Job drawing, mm, ordinate dimensions from the low corner. One solid piece. A direction names the side the tool comes from. Round coordinates to 2 decimals unless told otherwise and drop trailing zeros. Loops run counter-clockwise (first coordinate to the right, second up) from the corner with the lowest first, then second, coordinate; pieces in that order, holes last. Notation, with made-up numbers: M 78.25,-4.75 L 105.25,-4.75 A24 cw 105.25,13.25 Z; hole C 13.25,46.25 d5. An arc over 180 degrees is marked long. Use a Markdown table: item, result. Add a question column.
(1) Band-saw the part on C-C, the plane x = 44.5. Write the cut outline in (y, z), and give its area (3 significant figures).
(2) Band-saw the part on B-B, the plane y = 31. Write the cut outline in (x, z), and give its area (3 significant figures).
(3) Band-saw the part on D-D, the plane y = 59. Write the cut outline in (x, z).
(4) Which spindle directions (+Z, -Z, +X, -X, +Y, -Y) get a long thin tool onto all of the face, cutting with end or side? Do the marked faces 4, 5, 6 and 7. Say none if no direction does.
(5) Two-plate mould, pull along X, no slides. Class the marked faces 1, 2 and 3: released by +X, released by -X, zero draft, split by the parting line, or undercut.
(6) Flat gauge pins, fed straight in: P1, Ø10, axis at x = 17, z = 11, coming from the +Y side; P2, Ø1.5, axis at x = 27, y = 43, coming from the +Z side; P3, Ø12.5, axis at x = 35, z = 29.5, coming from the +Y side. Where does each tip first touch, or does it go through?
(7) Band-saw the part on A-A, the plane z = 42. Write the cut outline in (x, y).
(8) Wall check: L1, parallel to Y at x = 98.5, z = 44; L2, parallel to Y at x = 10.5, z = 35; L3, parallel to X at y = 28, z = 20. Give the ranges that are in metal, low to high.
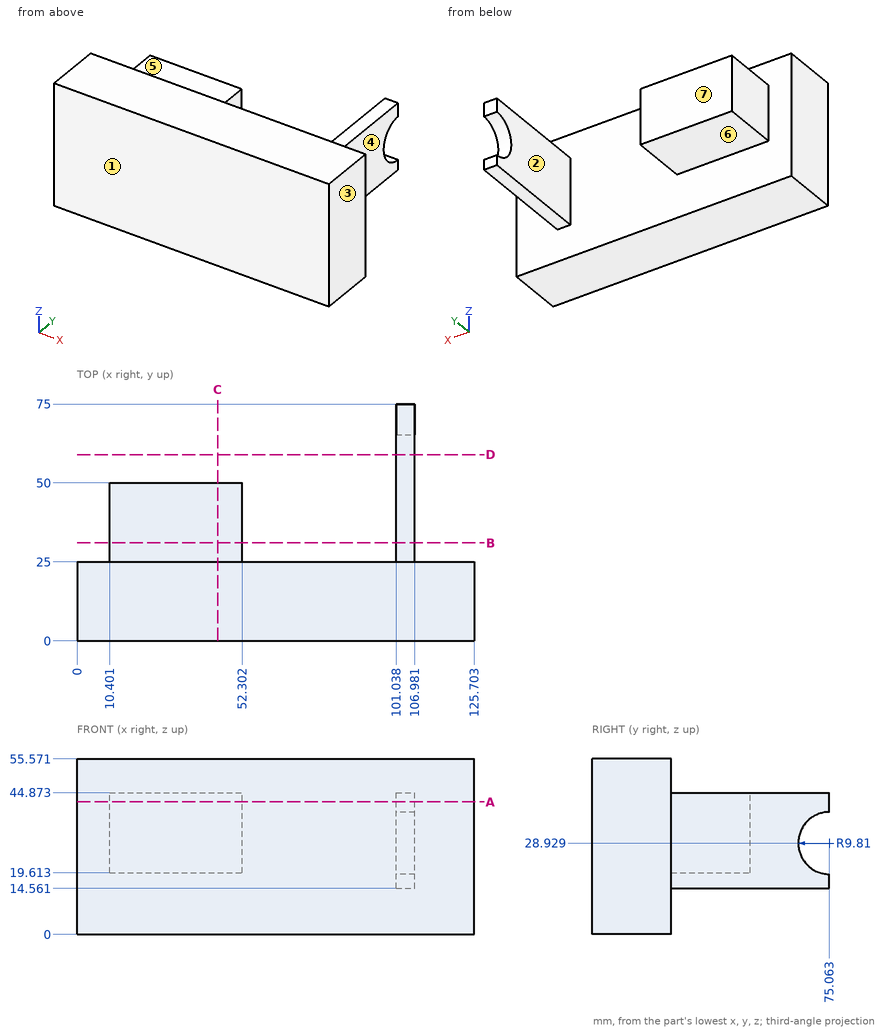
Return value:
| question | item | result |
|---|---|---|
| 1 | outline | M 0,0 L 25,0 L 25,19.61 L 50,19.61 L 50,44.87 L 25,44.87 L 25,55.57 L 0,55.57 Z |
| 1 | area | 2,020 mm^2 |
| 2 | outline | M 10.4,19.61 L 52.3,19.61 L 52.3,44.87 L 10.4,44.87 Z; M 101.04,14.56 L 106.98,14.56 L 106.98,44.87 L 101.04,44.87 Z |
| 2 | area | 1,240 mm^2 |
| 3 | outline | M 101.04,14.56 L 106.98,14.56 L 106.98,44.87 L 101.04,44.87 Z |
| 4 | face 4 | +Z, -Z, +X, +Y |
| 4 | face 5 | +Z, +X, -X, +Y |
| 4 | face 6 | -Z, -X, +Y |
| 4 | face 7 | +Z, -Z, -X, +Y |
| 5 | face 1 | zero draft |
| 5 | face 2 | undercut |
| 5 | face 3 | released by +X |
| 6 | P1 | y = 25 |
| 6 | P2 | z = 44.87 |
| 6 | P3 | y = 50 |
| 7 | outline | M 0,0 L 125.7,0 L 125.7,25 L 106.98,25 L 106.98,75 L 101.04,75 L 101.04,25 L 52.3,25 L 52.3,50 L 10.4,50 L 10.4,25 L 0,25 Z |
| 8 | L1 | 0 to 25 |
| 8 | L2 | 0 to 50 |
| 8 | L3 | 10.4 to 52.3, 101.04 to 106.98 |
